The listing builds one solid part. Answer for the finished solid, in the listing's coordinates (mm). Face numbers are marked on the shaded views. A direction names the side the tool comes from. Give positions to 0.01 mm unless a question says otherwise; leave off trailing zeros. Loops run counter-clockwise (first coordinate to the right, second up) from the corner with the lowest first, then second, coordinate; pieces in that order, holes last. Notation, with made-up numbers: (88, 48.25) - (146, 48.25) arc R29 ccw to (146, 69.25) - close; hole circle Ø2 at (77.5, -25). An arc over 180 degrees is marked (long way). Answer as CSV lines item,"result". Start each with the question number.
1) A cutting plane is placed at B-B (z = -559.5). Determine the outline of the cut face in (x, y) (3 decimals).
2) For a pull along X with two mould halves and no side action, classify the marked faces 1, 2, 3 and 4 as pulls with the +X half, pulls with the -X half, needs draft (parallel to the pull), parting line crosses it, or undercut.
3) A cutting plane is placed at D-D (z = -83.5). Determine the outline of the cut face in (x, y) (3 decimals), and give its area (3 significant figures).
4) A cutting plane is placed at A-A (y = 185). Give the number of separate pieces and of enclosed holes in the cut face, and give its area (3 significant figures).
5) A flat-ended cylindrical pin translates along its axis: pin 1 (4 mm diameter, centred on x = 806.5, z = -338.5, fed in from -Y). Find the tip coordinate at first contact, or state that the pin passes through.
6) A cutting plane is placed at C-C (x = 179.5). Determine the outline of the cut face in (y, z) (3 decimals), and give its area (3 significant figures).
7) For the marked faces 5 and 6, determine the directions among +Z, -Z, +X, -X, +Y, -Y from which every point of the face is accessible in a straight line to the end or side of a thin tool.
8) Find the intervals of material crossed by line 1 along Z through (x, y) = (923, 287); line 2 along X through (y, z) = (318, -294); line 3 along X through (y, z) = (154.5, -485.5), in increasing order.
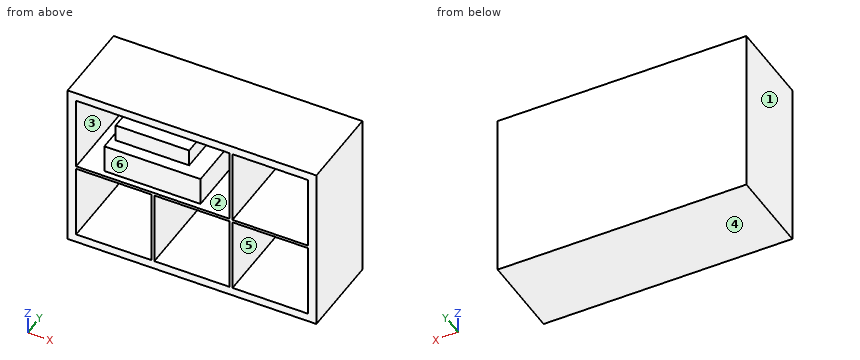
```python
from build123d import *

# Parameters (mm, degrees)
F0_W     = 1117.6
F0_H     = 762
F0_W_2   = 338.666667
F0_H_2   = 336.55
F0_W_3   = 338.666666
F1_DEPTH = 381
F2_W     = 1117.6
F2_H     = 762
F3_DEPTH = 3.175
F4_W     = 330.2
F4_H     = 76.2
F4_W_2   = 431.8
F4_H_2   = 127
F5_DEPTH = 381


with BuildPart() as f1:
    # F0 (on Front) → F1 (new body)
    with BuildSketch(Plane.XZ):
        with Locations((558.8, -381)):
            Rectangle(F0_W, F0_H)
        with Locations((207.433334, -555.625)):
            Rectangle(F0_W_2, F0_H_2, mode=Mode.SUBTRACT)
        with Locations((558.8, -555.625)):
            Rectangle(F0_W_3, F0_H_2, mode=Mode.SUBTRACT)
        with Locations((910.166667, -555.625)):
            Rectangle(F0_W_2, F0_H_2, mode=Mode.SUBTRACT)
        Polygon((38.1, -374.65), (38.1, -38.1), (376.766667, -38.1), (389.466667, -38.1), (728.133333, -38.1), (728.133333, -374.65), (389.466667, -374.65), (376.766667, -374.65), align=None, mode=Mode.SUBTRACT)
        with Locations((910.166667, -206.375)):
            Rectangle(F0_W_2, F0_H_2, mode=Mode.SUBTRACT)
    extrude(amount=-F1_DEPTH)

    # F2 (on face) → F3 (join)
    with BuildSketch(Plane(origin=(0, 381, 0), x_dir=(-1, 0, 0), z_dir=(0, 1, 0))):
        with Locations((-558.8, -381)):
            Rectangle(F2_W, F2_H)
    extrude(amount=F3_DEPTH)

    # F4 (on Front) → F5 (join)
    with BuildSketch(Plane.XZ):
        with Locations((381, -133.35)):
            Rectangle(F4_W, F4_H)
        with Locations((381, -285.75)):
            Rectangle(F4_W_2, F4_H_2)
    extrude(amount=-F5_DEPTH)


solid = f1.part
```
Ans:
1,outline,"(0, 0) - (38.1, 0) - (38.1, 381) - (376.767, 381) - (376.767, 0) - (389.467, 0) - (389.467, 381) - (728.133, 381) - (728.133, 0) - (740.833, 0) - (740.833, 381) - (1079.5, 381) - (1079.5, 0) - (1117.6, 0) - (1117.6, 384.175) - (0, 384.175) - close"
2,face 1,"pulls with the -X half"
2,face 2,"undercut"
2,face 3,"undercut"
2,face 4,"needs draft"
3,outline,"(0, 0) - (38.1, 0) - (38.1, 381) - (728.133, 381) - (728.133, 0) - (740.833, 0) - (740.833, 381) - (1079.5, 381) - (1079.5, 0) - (1117.6, 0) - (1117.6, 384.175) - (0, 384.175) - close"
3,area,"37,400 mm2"
4,separate pieces,"3"
4,enclosed holes,"5"
4,area,"243,000 mm2"
5,pin 1,"y = 381"
6,outline,"(0, -762) - (384.175, -762) - (384.175, 0) - (0, 0) - (0, -38.1) - (381, -38.1) - (381, -222.25) - (0, -222.25) - (0, -349.25) - (381, -349.25) - (381, -374.65) - (0, -374.65) - (0, -387.35) - (381, -387.35) - (381, -723.9) - (0, -723.9) - close"
6,area,"84,700 mm2"
7,face 5,"-Y"
7,face 6,"+Z, -Z, +X, -X, -Y"
8,line 1,"-762 to -723.9, -387.35 to -374.65, -38.1 to 0"
8,line 2,"0 to 38.1, 165.1 to 596.9, 728.13 to 740.83, 1079.5 to 1117.6"
8,line 3,"0 to 38.1, 376.77 to 389.47, 728.13 to 740.83, 1079.5 to 1117.6"
